Read the model definition and answer for the solid it produces. Units are mm, in the model's axes. Round coordinates to 2 decimals unless told otherwise and drop trailing zeros. Write each loop counter-clockwise with the first axis right and the second up, starting at its lowest first coordinate (ties: lowest second). Pieces come first, ordered by that corner, then holes. Notation, with made-up numbers: (-8, 66) - (42, 66) arc R23 cw to (42, 100) - close; hole circle Ø7 at (23.5, 84). An arc over 180 degrees is marked (long way). One line per item, written item: value. Start each with the question number.
(1) Find the intervals of material crossed by L1, parallel to X at y = 637, z = 16.25; L2, parallel to Z at x = -90.5, y = 906.5, in increasing order.
(2) A cutting plane is placed at A-A, the plane y = 1044. Determine the outline of the cut face in (x, z).
(3) A cutting plane is placed at B-B, the plane z = 16. Determine the outline of the cut face in (x, y).
(4) Flat-ended cylindrical pins translate along their axes: pin 1 Ø6.5 at (y, z) = (954.5, 22) entering from -X; pin 2 Ø3 at (x, z) = (61, 23.5) entering from -Y; pin 3 Ø9.5 at (x, y) = (-100, 819) entering from +Z; pin 4 Ø8 at (y, z) = (252, 21.5) entering from +X. Find the tip coordinate at first contact, or state that the pin passes through.
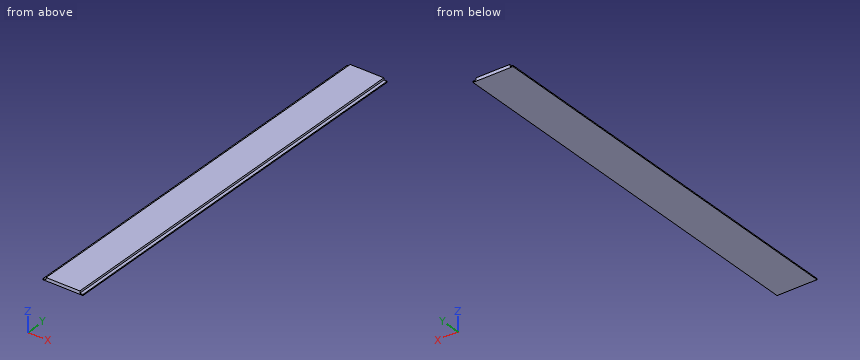
from build123d import *

# Parameters (mm, degrees)
F0_W     = 203.2
F0_H     = 12.7
F1_DEPTH = 2438.4


with BuildPart() as f1:
    # F0 (on Front) → F1 (new body)
    with BuildSketch(Plane.XZ):
        with Locations((14.341989, 19.369072)):
            Rectangle(F0_W, F0_H)
        Polygon((115.941989, 13.019072), (-87.258011, 13.019072), (-106.308011, 13.019072), (-106.308011, 6.669072), (134.991989, 6.669072), (134.991989, 13.019072), align=None)
    extrude(amount=-F1_DEPTH)


solid = f1.part
Here are the results:
1. L1: -87.26 to 115.94
1. L2: 6.67 to 13.02
2. outline: (-106.31, 6.67) - (134.99, 6.67) - (134.99, 13.02) - (115.94, 13.02) - (115.94, 25.72) - (-87.26, 25.72) - (-87.26, 13.02) - (-106.31, 13.02) - close
3. outline: (-87.26, 0) - (115.94, 0) - (115.94, 2438.4) - (-87.26, 2438.4) - close
4. pin 1: x = -87.26
4. pin 2: y = 0
4. pin 3: z = 13.02
4. pin 4: x = 115.94
